```python
from build123d import *

# Parameters (mm, degrees)
SKETCH1_W           = 30
SKETCH1_H           = 40
BOSS_EXTRUDE1_DEPTH = 8
SKETCH2_W           = 30
SKETCH2_H           = 8
BOSS_EXTRUDE2_DEPTH = 20
SKETCH3_R           = 2.5
CUT_EXTRUDE1_DEPTH  = 10
SKETCH4_R           = 2.5
CUT_EXTRUDE2_DEPTH  = 10
FILLET2_R           = 10


with BuildPart() as part:
    # Sketch1 → Boss-Extrude1 (new body)
    with BuildSketch(Plane(origin=(0, 0, 0), x_dir=(1, 0, 0), z_dir=(0, 1, 0))):
        with Locations((15, 20)):
            Rectangle(SKETCH1_W, SKETCH1_H)
    extrude(amount=BOSS_EXTRUDE1_DEPTH)

    # Sketch2 → Boss-Extrude2 (add)
    with BuildSketch(Plane.XZ):
        with Locations((15, -36)):
            Rectangle(SKETCH2_W, SKETCH2_H)
    extrude(amount=BOSS_EXTRUDE2_DEPTH)

    # Sketch3 → Cut-Extrude1 (cut)
    with BuildSketch(Plane(origin=(0, 8, 0), x_dir=(1, 0, 0), z_dir=(0, 1, 0))):
        with Locations((15, 11)):
            Circle(SKETCH3_R)
    extrude(amount=-CUT_EXTRUDE1_DEPTH, mode=Mode.SUBTRACT)

    # Sketch4 → Cut-Extrude2 (cut)
    with BuildSketch(Plane(origin=(0, 0, -40), x_dir=(-1, 0, 0), z_dir=(0, 0, -1))):
        with Locations((-15, -12)):
            Circle(SKETCH4_R)
    extrude(amount=-CUT_EXTRUDE2_DEPTH, mode=Mode.SUBTRACT)

    # Fillet2
    fillet2_edges = [part.edges().sort_by_distance(p)[0] for p in [
        (0, -20, -36),
        (30, -20, -36),
        (30, 4, 0),
        (0, 4, 0),
    ]]
    fillet(fillet2_edges, radius=FILLET2_R)


solid = part.part
```
The listing builds one solid part. Answer for the finished solid, in the listing's coordinates (mm). A direction names the side the tool comes from. Coordinates: 2 decimals unless noted, no trailing zeros. Loops run counter-clockwise (first coordinate to the right, second up) from the corner with the lowest first, then second, coordinate; pieces in that order, holes last. Notation, with made-up numbers: M -20.75,-13.75 L 16.25,-13.75 A17 cw 16.25,14.25 Z; hole C 7,53 d11. An arc over 180 degrees is marked long. Answer as a JSON object with one key per item and string values. Group by question number.
Item 1: Each of these flat-tipped pins is pushed along its axis until it touches: P1, Ø10, axis at x = 14, z = -9.5, coming from the -Y side; P2, Ø5, axis at x = 7, y = -12, coming from the +Z side. Where does it stop, or does it pass through?
Item 2: Section B-B (z = -11) is taken. Write down the section's boundary in (x, y), and give its area (3 significant figures).
Item 3: Section D-D (z = -4) is taken. Write down the section's boundary in (x, y), and give its area (3 significant figures).
Item 4: Determine the mould class of faces 1 (the face through (2.85, 4.06, -3.01)), 2 (the face through (13, 4.1, -9.5)), 3 (the face through (15, -20, -36)) for opening direction X: +X half, -X half, draft (parallel to the pull), parting line (faces both ways), or undercut.
Item 5: Section C-C (y = -12) is taken. Write down the section's boundary in (x, z).
Item 6: Consider L1, parallel to X at y = 5, z = -11; L2, parallel to Z at x = 15, y = 6; L3, parallel to Y at x = 15, z = -37. Determine where each line is inside the solid, lowest interval first.
Item 7: Which of the six approach directions +Z, -Z, +X, -X, +Y, -Y give full straight-line access (tool end or side, diameter ignored) to faces 4 (the face through (0, 3, -29)), 5 (the face through (15, 0, -16))?
Item 8: Section A-A (x = 13.5) is taken. Write down the section's boundary in (y, z), and give its area (3 significant figures).
Solved:
{
 "1": {"P1": "stops at y = 0", "P2": "stops at z = -32"},
 "2": {"outline": "M 0,0 L 12.5,0 L 12.5,8 L 0,8 Z; M 17.5,0 L 30,0 L 30,8 L 17.5,8 Z", "area": "200 mm2"},
 "3": {"outline": "M 2,0 L 28,0 L 28,8 L 2,8 Z", "area": "208 mm2"},
 "4": {"face 1": "-X half", "face 2": "undercut", "face 3": "draft"},
 "5": {"outline": "M 0.2,-40 L 12.5,-40 L 12.5,-32 L 0.2,-32 Z; M 17.5,-40 L 29.8,-40 L 29.8,-32 L 17.5,-32 Z"},
 "6": {"L1": "x = 0 to 12.5, 17.5 to 30", "L2": "z = -40 to -13.5, -8.5 to 0", "L3": "y = -20 to -14.5, -9.5 to 8"},
 "7": {"face 4": "+Z, -Z, -X, +Y, -Y", "face 5": "+Z, +X, -X, -Y"},
 "8": {"outline": "M -20,-40 L -14,-40 L -14,-32 L -20,-32 Z; M -10,-40 L 8,-40 L 8,-13 L 0,-13 L 0,-32 L -10,-32 Z; M 0,-9 L 8,-9 L 8,0 L 0,0 Z", "area": "416 mm2"}
}
